Source: three-view drawing plus pictorial views. Frame: mm from the lowest corner of the part. A direction names the side the tool comes from. Coordinates: 2 decimals unless noted, no trailing zeros. Write each loop counter-clockwise with the first axis right and the second up, starting at its lowest first coordinate (ties: lowest second). Pieces come first, ordered by that corner, then holes. Notation, with made-up numbers: M -12.75,-5 L 25.25,-5 A13 cw 25.25,19 Z; hole C -17,71.5 d6. An arc over 180 degrees is marked long. Answer as a JSON object with one key per item and string values. Group by question number.
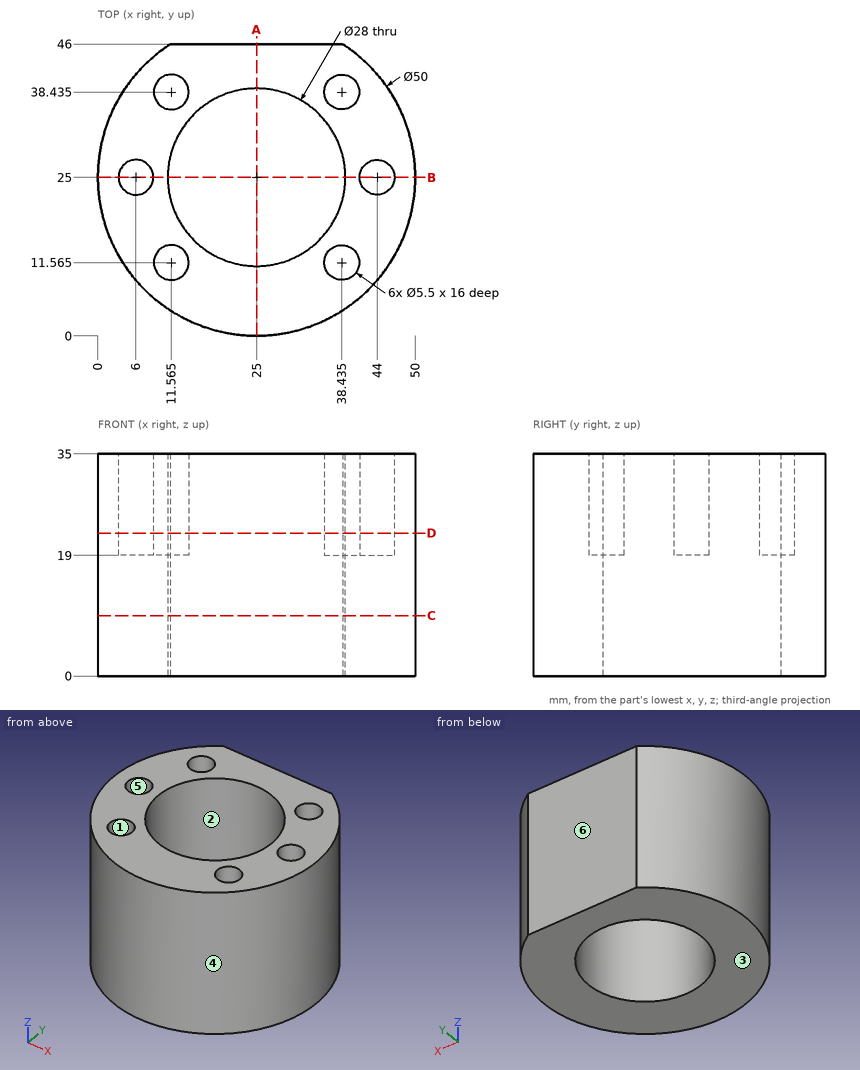
Q1. Draft query along Y for the marked faces 3, 4, 5 and 6. Return one class per face: released by +Y, released by -Y, zero draft, split by the parting line, or undercut.
Q2. Line query: line 1 (Y direction, x = 25, z = 24); line 2 (Y direction, x = 44, z = 24); line 3 (Y direction, x = 10.5, z = 29). Output: solid intervals per line, ascending. Write a range as from..to.
Q3. Access query for the marked faces 1 and 2. Directions: +Z, -Z, +X, -X, +Y, -Y. A direction counts if a zero-diameter tool reaches every point of the face in a straight line with its end or side. Return the directions, or none.
Q4. Section D-D, the plane z = 22.5. Return the cut outline in (x, y) (3 decimals), and give its area (3 significant figures).
Q5. Pin query (flat end, axial travel): pin 1 Ø1.6 at (x, y) = (38.5, 11) entering from +Z; pin 2 Ø6 at (x, z) = (34, 27) entering from -Y; pin 3 Ø4 at (y, z) = (7, 6) entering from -X. Return the tip coordinate at first contact, or that it passes through.
Q6. Section C-C, the plane z = 9.5. Return the cut outline in (x, y).
Q7. Section A-A, the plane x = 25. Return the cut outline in (y, z).
Q8. Section B-B, the plane y = 25. Return the cut outline in (x, z), and give its area (3 significant figures).
Filled in:
{
 "1": {"face 3": "zero draft", "face 4": "split by the parting line", "face 5": "undercut", "face 6": "released by +Y"},
 "2": {"line 1": "0..11, 39..46", "line 2": "8.75..22.25, 27.75..41.25", "line 3": "4.63..9.03, 14.1..35.9, 40.97..45.37"},
 "3": {"face 1": "+Z", "face 2": "+Z, -Z"},
 "4": {"outline": "M 11.435,46 A25 ccw long 38.565,46 Z; hole C 6,25 d5.5; hole C 11.565,11.565 d5.5; hole C 11.565,38.435 d5.5; hole C 25,25 d28; hole C 38.435,11.565 d5.5; hole C 38.435,38.435 d5.5; hole C 44,25 d5.5", "area": "1,130 mm^2"},
 "5": {"pin 1": "z = 19", "pin 2": "y = 0.73", "pin 3": "x = 5.79"},
 "6": {"outline": "M 11.44,46 A25 ccw long 38.56,46 Z; hole C 25,25 d28"},
 "7": {"outline": "M 0,0 L 11,0 L 11,35 L 0,35 Z; M 39,0 L 46,0 L 46,35 L 39,35 Z"},
 "8": {"outline": "M 0,0 L 11,0 L 11,35 L 8.75,35 L 8.75,19 L 3.25,19 L 3.25,35 L 0,35 Z; M 39,0 L 50,0 L 50,35 L 46.75,35 L 46.75,19 L 41.25,19 L 41.25,35 L 39,35 Z", "area": "594 mm^2"}
}
